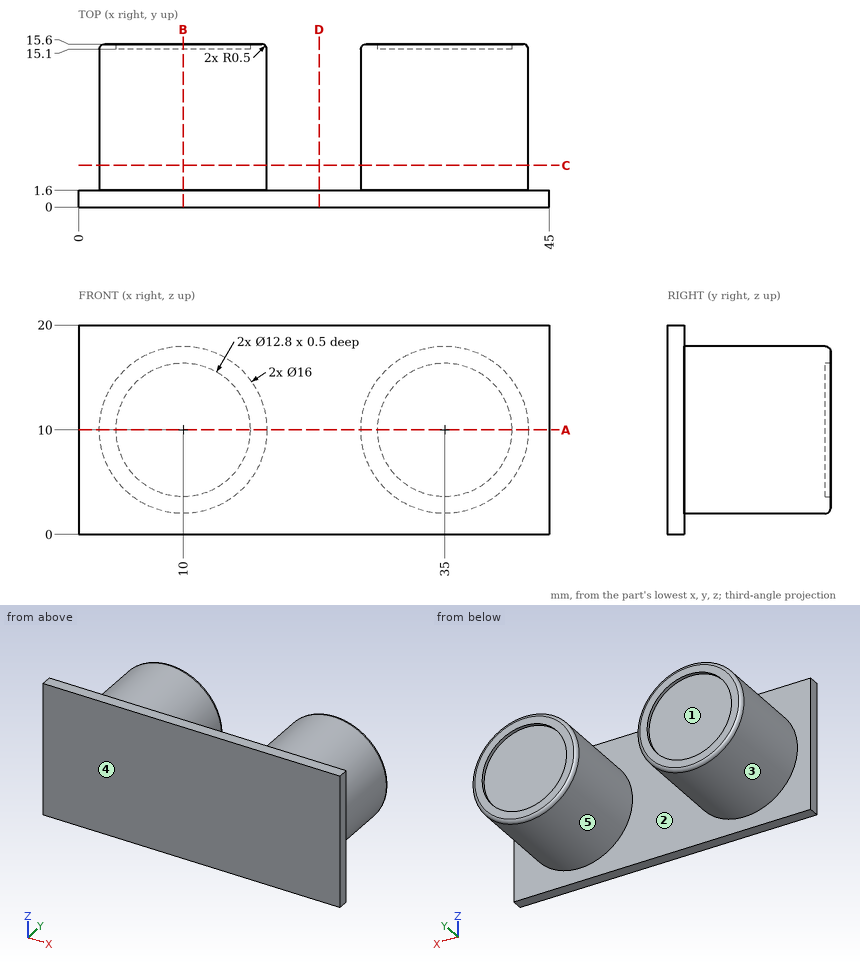
Here's the drawing with two shaded views (mm, measured from the low corner). I have some questions. A direction names the side the tool comes from. Round coordinates to 2 decimals unless told otherwise and drop trailing zeros. Loops run counter-clockwise (first coordinate to the right, second up) from the corner with the lowest first, then second, coordinate; pieces in that order, holes last. Notation, with made-up numbers: (20.25, 60.5) - (59.25, 60.5) arc R19 ccw to (59.25, 64.5) - close; hole circle Ø11 at (84, -22.5). An arc over 180 degrees is marked (long way). Write item = value, one per line.
1) Imagine slicing it at C-C (y = 4). Please give me the cut outline in (x, z), and give its area (3 significant figures).
Computed:
outline = circle Ø16 at (10, 10); circle Ø16 at (35, 10)
area = 402 mm2
2) Imagine slicing it at B-B (x = 10). Please give me the cut outline in (y, z).
Computed:
outline = (0, 0) - (1.6, 0) - (1.6, 2) - (15.1, 2) arc R0.5 ccw to (15.6, 2.5) - (15.6, 3.6) - (15.1, 3.6) - (15.1, 16.4) - (15.6, 16.4) - (15.6, 17.5) arc R0.5 ccw to (15.1, 18) - (1.6, 18) - (1.6, 20) - (0, 20) - close
3) Imagine slicing it at D-D (x = 23). Please give me the cut outline in (y, z), and give its area (3 significant figures).
Computed:
outline = (0, 0) - (1.6, 0) - (1.6, 20) - (0, 20) - close
area = 32.0 mm2
4) I need wall thicknesses on line 1 along X through (y, z) = (15.3, 10); line 2 along Y through (x, z) = (43.5, 7); line 3 along Y through (x, z) = (8, 16). Which ranges of each line are inside material? Lowest first, please. Write a range as from..to.
Computed:
line_1 = 2.04..3.6, 16.4..17.96, 27.04..28.6, 41.4..42.96
line_2 = 0..1.6
line_3 = 0..15.1
5) On a 3-axis mill with a long thin cutter (end or side, diameter ignored), from which of +Z, -Z, +X, -X, +Y, -Y can I reach the whole of each face in a straight line? I mean the marked faces 4 and 5. Say none if no direction works.
Computed:
face_4 = +Z, -Z, +X, -X, -Y
face_5 = +Y
6) I'm going to push flat-ended pins straight in: P1, Ø1, axis at x = 9.5, y = 9.5, coming from the +Z side; P2, Ø6, axis at y = 13, z = 15, coming from the +X side; P3, Ø2, axis at x = 24, z = 15.5, coming from the +Y side. Where does each tip first touch, or does it pass through?
Computed:
P1 = 18
P2 = 42.75
P3 = 1.6
7) Imagine slicing it at A-A (z = 10). Please give me the cut outline in (x, y).
Computed:
outline = (0, 0) - (45, 0) - (45, 1.6) - (43, 1.6) - (43, 15.1) arc R0.5 ccw to (42.5, 15.6) - (41.4, 15.6) - (41.4, 15.1) - (28.6, 15.1) - (28.6, 15.6) - (27.5, 15.6) arc R0.5 ccw to (27, 15.1) - (27, 1.6) - (18, 1.6) - (18, 15.1) arc R0.5 ccw to (17.5, 15.6) - (16.4, 15.6) - (16.4, 15.1) - (3.6, 15.1) - (3.6, 15.6) - (2.5, 15.6) arc R0.5 ccw to (2, 15.1) - (2, 1.6) - (0, 1.6) - close
8) If we mould it in two halves opening along Z, with no side actions, what happens to the marked faces 1, 2 and 3? For each: pulls with the +Z half, pulls with the -Z half, needs draft (parallel to the pull), parting line crosses it, or undercut.
Computed:
face_1 = undercut
face_2 = needs draft
face_3 = parting line crosses it
